```python
from build123d import *

# Parameters (mm, degrees)
F0_R         = 1.75
F1_DEPTH     = 5
F2_R         = 3
F3_DEPTH     = 3
F4_T1_DEPTH  = 23.0280702819
F4_T3_DEPTH  = 26.0887631675
F4_T5_DEPTH  = 26.0887631675
F4_T8_ANGLE  = 116.1894596418
F4_T10_ANGLE = 116.1894596418
F4_T12_ANGLE = 127.6210807165


# Not quite as in the source:
# - a fillet or chamfer that OpenCascade refuses, or shapes differently, is made with other operations: its cross-section is extruded or revolved along the edge and cut away or added


with BuildPart() as f1:
    # F0 (on Top) → F1 (new body)
    with BuildSketch(Plane.XY):
        with BuildLine():
            Line((6.1053208487, 22.0431612343), (-5.4087142923, -1.3673184358))
            ThreePointArc((-5.4087142923, -1.3673184358), (-5.3118812954, -3.3070328452), (-3.6140351409, -4.25))
            Line((-3.6140351409, -4.25), (19.4140351409, -4.25))
            ThreePointArc((19.4140351409, -4.25), (21.1118812954, -3.3070328452), (21.2087142923, -1.3673184358))
            Line((21.2087142923, -1.3673184358), (9.6946791513, 22.0431612343))
            ThreePointArc((9.6946791513, 22.0431612343), (7.9, 23.16047967), (6.1053208487, 22.0431612343))
        make_face()
        Circle(F0_R, mode=Mode.SUBTRACT)
        with Locations((15.8, 0)):
            Circle(F0_R, mode=Mode.SUBTRACT)
        with Locations((7.9, 16.0623784042)):
            Circle(F0_R, mode=Mode.SUBTRACT)
    extrude(amount=F1_DEPTH)

    # F2 (on Top) → F3 (cut)
    with BuildSketch(Plane.XY):
        with Locations((15.8, 0)):
            Circle(F2_R)
        Circle(F2_R)
        with Locations((7.9, 16.0623784042)):
            Circle(F2_R)
    extrude(amount=F3_DEPTH, mode=Mode.SUBTRACT)

    # F4: chamfer of 2 on 1 edges, made by hand

    # F4_s2 → F4_t1 (cut)
    with BuildSketch(Plane.YZ.offset(-3.6140351409)):
        Polygon((-2.25, 0), (-4.25, 2), (-4.25, 0), align=None)
    extrude(amount=F4_T1_DEPTH, mode=Mode.SUBTRACT)

    # F4_s4 → F4_t3 (cut)
    with BuildSketch(Plane(origin=(4.672571734, -9.5003310521, 0), x_dir=(0, 0, 1), z_dir=(-0.4413407821, 0.8973395757, 0))):
        Polygon((2, 18.4279652953), (0, 16.4279652953), (0, 18.4279652953), align=None)
    extrude(amount=F4_T3_DEPTH, mode=Mode.SUBTRACT)

    # F4_s6 → F4_t5 (cut)
    with BuildSketch(Plane(origin=(9.9190140452, 20.1674629103, 0), x_dir=(0, 0, 1), z_dir=(-0.4413407821, -0.8973395757, 0))):
        Polygon((2, 4.25), (0, 2.25), (0, 4.25), align=None)
    extrude(amount=F4_T5_DEPTH, mode=Mode.SUBTRACT)

    # F4_s7 → F4_t8 (revolve, cut)
    with BuildSketch(Plane(origin=(-1.5950210957, -3.2430167598, 0), x_dir=(0, 0, 1), z_dir=(0.4413407821, 0.8973395757, 0))):
        Polygon((0, -2.25), (2, -4.25), (0, -4.25), align=None)
    revolve(axis=Axis((-3.6140351409, -2.25, 0), (0, 0, 1)), revolution_arc=F4_T8_ANGLE, mode=Mode.SUBTRACT)

    # F4_s9 → F4_t10 (revolve, cut)
    with BuildSketch(Plane.YZ.offset(19.4140351409)):
        Polygon((-2.25, 0), (-4.25, 2), (-4.25, 0), align=None)
    revolve(axis=Axis((19.4140351409, -2.25, 0), (0, 0, 1)), revolution_arc=F4_T10_ANGLE, mode=Mode.SUBTRACT)

    # F4_s11 → F4_t12 (revolve, cut)
    with BuildSketch(Plane(origin=(-6.841463407, 13.9101486179, 0), x_dir=(0, 0, 1), z_dir=(0.4413407821, -0.8973395757, 0))):
        Polygon((2, -18.4279652953), (0, -16.4279652953), (0, -18.4279652953), align=None)
    revolve(axis=Axis((7.9, 21.16047967, 0), (0, 0, 1)), revolution_arc=F4_T12_ANGLE, mode=Mode.SUBTRACT)


solid = f1.part
```
The model under review builds one solid part; all positions refer to its coordinate system, in mm. A direction names the side the tool comes from. Round coordinates to 2 decimals unless told otherwise and drop trailing zeros. Order: outer loops, then holes, each group sorted by start corner. A loop starts at its lowest first (then second) coordinate and runs counter-clockwise, first axis right, second up. Notation, with made-up numbers: (-13, 70) -> (29, 70) arc R31 cw to (29, 103) -> close; hole circle Ø6 at (20, -35). An arc over 180 degrees is marked (long way). One line per item, written item: value. Start each with the question number.
Q1. Wall thickness on line 1 (Y direction, x = 7.9, z = 3.6); line 2 (X direction, y = 0, z = 1); line 3 (X direction, y = 0, z = 3.95): over which ranges is each line inside the solid? List them lowest first.
Q2. Take a section at B-B (z = 3.4). Write out the cut boundary in (x, y), and give its area (3 significant figures).
Q3. Clearance check with flat-ended pins moving along their axes: pin 1 Ø3 at (y, z) = (11, 1) entering from -X; pin 2 Ø5 at (x, y) = (0, 16.5) entering from -Z; pin 3 Ø3 at (x, y) = (17, -0.5) entering from -Z; pin 4 Ø7 at (x, y) = (7.9, 16.06) entering from -Z. State where each tip first meets the part, or that it passes through.
Q4. Machinability: for faces 1 (the face through (7.74, -3.24, 0.99)), 2 (the face through (9.28, 13.4, 1.48)), which of the approach directions +Z, -Z, +X, -X, +Y, -Y give a long, thin tool a straight path to every point of the face, cutting with its end or side? Answer none if there is none.
Q5. Take a section at C-C (x = 0). Write out the cut boundary in (y, z), and give its area (3 significant figures).
Q6. Take a section at D-D (y = 7.5). Write out the cut boundary in (x, z), and give its area (3 significant figures).
Q7. Mouldability with a two-part tool opening along Y and no side actions: class faces 3 (the face through (-4.48, -2.77, 1.01)), 4 (the face through (8, 14, 3)), 5 (the face through (0, -2, 3)), 6 (the face through (-3, -2, 0)) as released by +Y, released by -Y, zero draft, split by the parting line, or undercut.
Q8. Take a section at A-A (y = 0). Write out the cut boundary in (x, z).
Reported:
1. line 1: y = -4.25 to 14.31, 17.81 to 23.16
1. line 2: x = -3.62 to -3, 3 to 12.8, 18.8 to 19.42
1. line 3: x = -4.74 to -1.75, 1.75 to 14.05, 17.55 to 20.54
2. outline: (-5.41, -1.37) arc R2 ccw to (-3.61, -4.25) -> (19.41, -4.25) arc R2 ccw to (21.21, -1.37) -> (9.69, 22.04) arc R2 ccw to (6.11, 22.04) -> close; hole circle Ø3.5 at (0, 0); hole circle Ø3.5 at (7.9, 16.06); hole circle Ø3.5 at (15.8, 0)
2. area: 404 mm2
3. pin 1: stops at x = 0.12
3. pin 2: passes through
3. pin 3: stops at z = 3
3. pin 4: stops at z = 0
4. face 1: -Z, +X, -X, -Y
4. face 2: -Z
5. outline: (-4.25, 2) -> (-3, 0.75) -> (-3, 3) -> (-1.75, 3) -> (-1.75, 5) -> (-4.25, 5) -> close; (1.75, 3) -> (3, 3) -> (3, 0) -> (5.1, 0) -> (9.63, 2) -> (9.63, 5) -> (1.75, 5) -> close
5. area: 38.1 mm2
6. outline: (-1.05, 2) -> (1.18, 0) -> (14.62, 0) -> (16.85, 2) -> (16.85, 5) -> (-1.05, 5) -> close
6. area: 85.0 mm2
7. face 3: split by the parting line
7. face 4: undercut
7. face 5: undercut
7. face 6: zero draft
8. outline: (-4.74, 2) -> (-3, 0.44) -> (-3, 3) -> (-1.75, 3) -> (-1.75, 5) -> (-4.74, 5) -> close; (1.75, 3) -> (3, 3) -> (3, 0) -> (12.8, 0) -> (12.8, 3) -> (14.05, 3) -> (14.05, 5) -> (1.75, 5) -> close; (17.55, 3) -> (18.8, 3) -> (18.8, 0.44) -> (20.54, 2) -> (20.54, 5) -> (17.55, 5) -> close
